Source: three-view drawing plus pictorial views. Frame: mm from the lowest corner of the part. A direction names the side the tool comes from. Coordinates: 2 decimals unless noted, no trailing zeros. Loops run counter-clockwise (first coordinate to the right, second up) from the corner with the lowest first, then second, coordinate; pieces in that order, holes last. Notation, with made-up numbers: M 72,-11.5 L 77,-11.5 A33 ccw 77,26.5 Z; hole C 78.25,-37.75 d7. An arc over 180 degrees is marked long. Use a Markdown table: item, result. Add a question column.
1. Set-up query: the marked faces 1, 2 and 3. Return all of +Z, -Z, +X, -X, +Y, -Y with unobstructed straight access to the full face (end or side cutting, diameter ignored); none if empty.
2. Section C-C on y = 30. Output: boundary loops of the cut face in (x, z).
3. Section D-D on z = 35.5. Output: boundary loops of the cut face in (x, y).
4. Section A-A on y = 8. State how many separate pieces and enclosed holes the cut face has, then the cut area to 3 significant figures.
5. Draft query along X for the marked faces 4, 5 and 6. Return one class per face: +X half, -X half, draft (parallel to the pull), parting line (faces both ways), or undercut.
6. Section B-B on z = 25.5. Output: boundary loops of the cut face in (x, y), then the cut area to 3 significant figures.
7. Pin query (flat end, axial travel): pin 1 (5 mm diameter, centred on x = 81.5, z = 9, fed in from +Y); pin 2 (1.5 mm diameter, centred on y = 5.5, z = 18.5, fed in from -X); pin 3 (3 mm diameter, centred on y = 13, z = 22.5, fed in from -X). Return the tip coordinate at first contact, or that it passes through.
8. Line query: L1, parallel to Y at x = 37, z = 19; L2, parallel to X at y = 6, z = 17.5; L3, parallel to X at y = 8.5, z = 19 (1 decimal). Output: solid intervals per line, ascending. Write a range as [from, to].
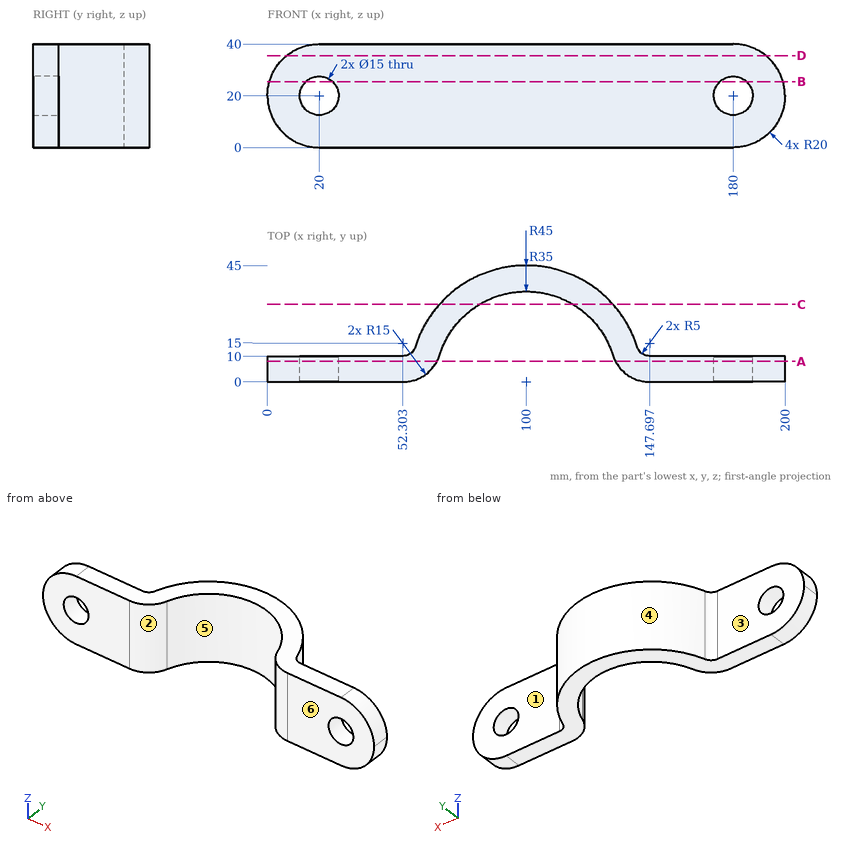
Answers below:
| question | item | result |
|---|---|---|
| 1 | face 1 | +Z, -Z, +X, +Y |
| 1 | face 2 | +Z, -Z, -Y |
| 1 | face 3 | +Z, -Z, -X, +Y |
| 2 | outline | M 66.46,0 L 81.97,0 L 81.97,40 L 66.46,40 Z; M 118.03,0 L 133.54,0 L 133.54,40 L 118.03,40 Z |
| 3 | outline | M 7.36,0 L 52.3,0 A15 ccw 66.61,10.5 A35 cw 133.39,10.5 A15 ccw 147.7,0 L 192.64,0 L 192.64,10 L 147.7,10 A5 cw 142.93,13.5 A45 ccw 57.07,13.5 A5 cw 52.3,10 L 7.36,10 Z |
| 4 | separate pieces | 2 |
| 4 | enclosed holes | 2 |
| 4 | area | 4,550 mm² |
| 5 | face 4 | parting line |
| 5 | face 5 | undercut |
| 5 | face 6 | draft |
| 6 | outline | M 0.77,0 L 14.9,0 L 14.9,10 L 0.77,10 Z; M 25.1,0 L 52.3,0 A15 ccw 66.61,10.5 A35 cw 133.39,10.5 A15 ccw 147.7,0 L 174.9,0 L 174.9,10 L 147.7,10 A5 cw 142.93,13.5 A45 ccw 57.07,13.5 A5 cw 52.3,10 L 25.1,10 Z; M 185.1,0 L 199.23,0 L 199.23,10 L 185.1,10 Z |
| 6 | area | 2,090 mm² |
| 7 | pin 1 | stops at y = 42.06 |
| 7 | pin 2 | stops at x = 0.01 |
| 7 | pin 3 | stops at x = 55.87 |
| 8 | L1 | y = [0, 10] |
| 8 | L2 | x = [0.16, 12.93], [27.07, 64.3], [135.7, 172.93], [187.07, 199.84] |
| 8 | L3 | x = [0, 12.6], [27.4, 65.8], [134.2, 172.6], [187.4, 200] |
